Answer from the drawing. Dimensions are ordinates in mm from the lowest x, y and z of the part. Round coordinates to 2 decimals unless told otherwise and drop trailing zeros. Write each loop counter-clockwise with the first axis right and the second up, starting at its lowest first coordinate (ties: lowest second). Pieces come first, ordered by that corner, then holes. Notation, with made-up numbers: (-18.5, 52) -> (27.5, 52) arc R8 cw to (27.5, 60) -> close; hole circle Ø6 at (71, 11). An arc over 180 degrees is marked (long way). Return JSON: item names as keys, results as strings. Group by question number.
(1) Given pin 1 (3 mm diameter, centred on y = 91.5, z = 12, fed in from +X); pin 2 (12 mm diameter, centred on x = 10, z = 24.5, fed in from -Y); pin 3 (10 mm diameter, centred on x = 22, y = 60.5, fed in from +Z); pin 4 (1.5 mm diameter, centred on x = 25.5, y = 82.5, fed in from -Z), each flat-ended and moving along its own axis, determine where each tip first touches the part or whether it passes through.
(2) Straight lines are drawn through the part: line 1 (Z direction, x = 14.7, y = 63); line 2 (Y direction, x = 28.25, z = 20.25); line 3 (Z direction, x = 18.75, y = 119). For each, find the intervals that lie inside material, in ascending order.
(3) A cutting plane is placed at A-A on z = 14.7. Give the vertices of the cut face in (x, y), then the cut area to 3 significant figures.
(4) A cutting plane is placed at B-B on x = 14.7. Give the vertices of the cut face in (y, z).
(5) A cutting plane is placed at C-C on y = 45. Give the vertices of the cut face in (x, z), then the cut area to 3 significant figures.
(6) The mould has two halves that part along X. Classify the marked faces 1 and 2: released by +X, released by -X, zero draft, split by the parting line, or undercut.
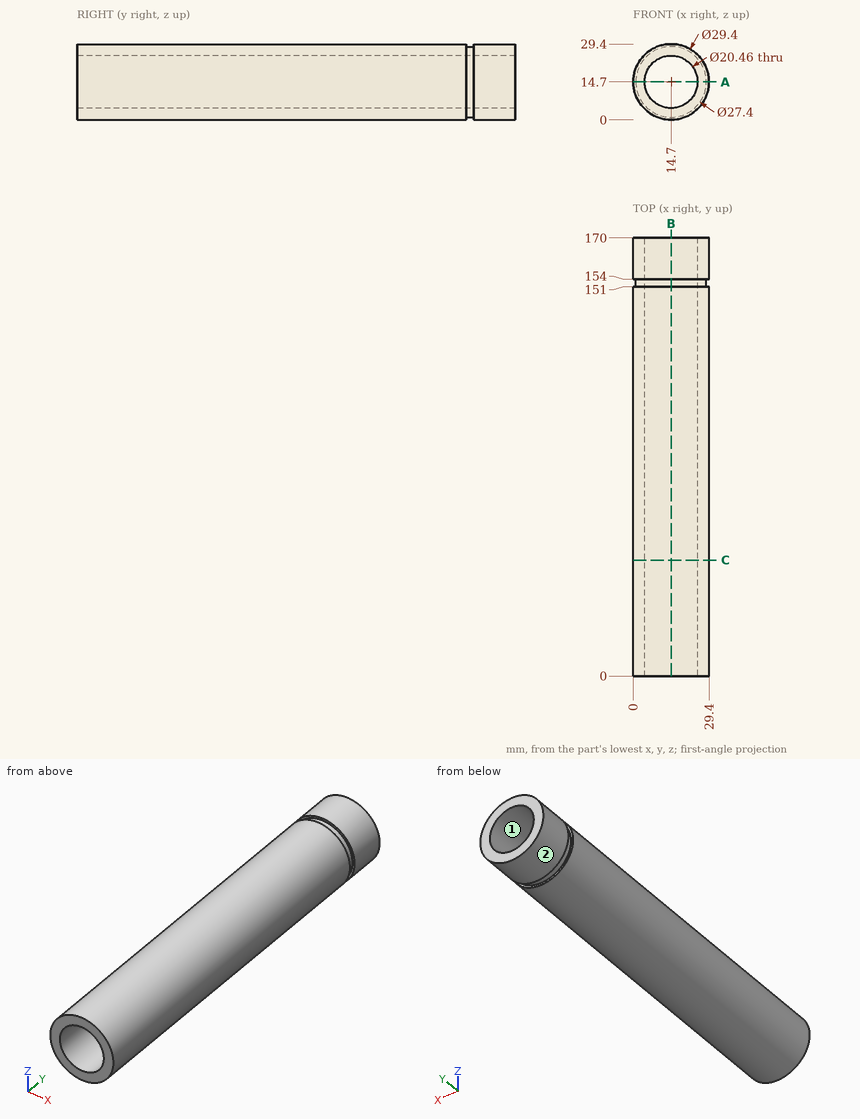
Checks:
{
 "1": {"pin 1": "stops at x = 29.35", "pin 2": "stops at y = 0", "pin 3": "stops at z = 29.22", "pin 4": "stops at z = 3.97"},
 "2": {"line 1": "z = 0 to 4.47, 24.93 to 29.4", "line 2": "y = 0 to 151, 154 to 170", "line 3": "z = 0.57 to 5.31, 24.09 to 28.83"},
 "3": {"outline": "(0, 0) -> (4.47, 0) -> (4.47, 170) -> (0, 170) -> (0, 154) -> (1, 154) -> (1, 151) -> (0, 151) -> close; (24.93, 0) -> (29.4, 0) -> (29.4, 151) -> (28.4, 151) -> (28.4, 154) -> (29.4, 154) -> (29.4, 170) -> (24.93, 170) -> close", "area": "1,510 mm^2"},
 "4": {"outline": "(0, 0) -> (151, 0) -> (151, 1) -> (154, 1) -> (154, 0) -> (170, 0) -> (170, 4.47) -> (0, 4.47) -> close; (0, 24.93) -> (170, 24.93) -> (170, 29.4) -> (154, 29.4) -> (154, 28.4) -> (151, 28.4) -> (151, 29.4) -> (0, 29.4) -> close"},
 "5": {"outline": "circle Ø29.4 at (14.7, 14.7); hole circle Ø20.46 at (14.7, 14.7)", "area": "350 mm^2"},
 "6": {"face 1": "undercut", "face 2": "split by the parting line"}
}
